CAD build for the part. Positions are in the model's coordinates, mm. Give positions to 0.01 mm unless a question says otherwise; leave off trailing zeros. Loops run counter-clockwise (first coordinate to the right, second up) from the corner with the lowest first, then second, coordinate; pieces in that order, holes last. Notation, with made-up numbers: (71.25, 10) - (105.25, 10) arc R28 cw to (105.25, 39) - close; hole circle Ø2 at (75, 70.5). An arc over 180 degrees is marked (long way). Return JSON: item names as keys, results as strings.
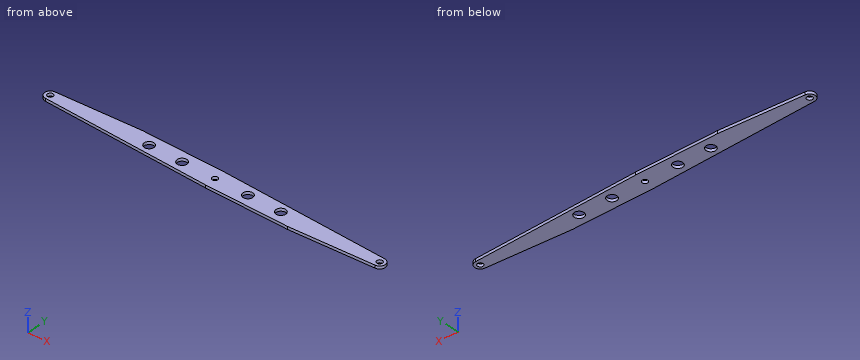
from build123d import *

# Parameters (mm, degrees)
SKETCH1_R           = 10
SKETCH1_R_2         = 17.5
BOSS_EXTRUDE1_DEPTH = 5


with BuildPart() as part:
    # Sketch1 → Boss-Extrude1 (new body, symmetric)
    with BuildSketch(Plane.XY):
        with BuildLine():
            Line((0, 40), (-300, 40))
            Line((-300, 40), (-601.327453078, 19.955898084))
            ThreePointArc((-601.327453078, 19.955898084), (-619.997257899, -0.331174458), (-600.665927363, -19.988910444))
            Line((-600.665927363, -19.988910444), (0, -40))
            Line((0, -40), (300, -40))
            Line((300, -40), (601.327453078, -19.955898084))
            ThreePointArc((601.327453078, -19.955898084), (619.997257899, 0.331174458), (600.665927363, 19.988910444))
            Line((600.665927363, 19.988910444), (0, 40))
        make_face()
        with Locations((-600, 0)):
            Circle(SKETCH1_R, mode=Mode.SUBTRACT)
        with Locations((600, 0)):
            Circle(SKETCH1_R, mode=Mode.SUBTRACT)
        Circle(SKETCH1_R, mode=Mode.SUBTRACT)
        with Locations((-120, 0)):
            Circle(SKETCH1_R_2, mode=Mode.SUBTRACT)
        with Locations((-240, 0)):
            Circle(SKETCH1_R_2, mode=Mode.SUBTRACT)
        with Locations((120, 0)):
            Circle(SKETCH1_R_2, mode=Mode.SUBTRACT)
        with Locations((240, 0)):
            Circle(SKETCH1_R_2, mode=Mode.SUBTRACT)
    extrude(amount=BOSS_EXTRUDE1_DEPTH, both=True)


solid = part.part
1. Drop flat-ended pins along their axis: P1, Ø4, axis at x = -422.5, z = -1.5, coming from the +Y side; P2, Ø3, axis at x = 333.5, z = 1, coming from the +Y side. Give the stop position or say it passes through.
Values follow:
{"P1": "stops at y = 31.98", "P2": "stops at y = 28.94"}
2. Cut at A-A, the plane z = -2.5. Write the cut outline in (x, y), plus the area to 3 significant figures.
Values follow:
{"outline": "(-601.33, 19.96) arc R20 ccw to (-600.67, -19.99) - (0, -40) - (300, -40) - (601.33, -19.96) arc R20 ccw to (600.67, 19.99) - (0, 40) - (-300, 40) - close; hole circle Ø20 at (-600, 0); hole circle Ø35 at (-240, 0); hole circle Ø35 at (-120, 0); hole circle Ø20 at (0, 0); hole circle Ø35 at (120, 0); hole circle Ø35 at (240, 0); hole circle Ø20 at (600, 0)", "area": "74,500 mm²"}
3. Cut at D-D, the plane x = -542. Write the cut outline in (y, z).
Values follow:
{"outline": "(-21.94, -5) - (23.9, -5) - (23.9, 5) - (-21.94, 5) - close"}
4. Cut at B-B, the plane x = 120. Write the cut outline in (y, z).
Values follow:
{"outline": "(-40, -5) - (-17.5, -5) - (-17.5, 5) - (-40, 5) - close; (17.5, -5) - (36, -5) - (36, 5) - (17.5, 5) - close"}
5. Drill centre lines: probe 1 along X at (y, z) = (11, -0.25); probe 2 along Y at (x, z) = (2, 3.25); probe 3 along X at (y, z) = (-11.5, -2.5). Where is each one in solid material? Low to high.
Values follow:
{"probe 1": "x = -616.7 to -253.61, -226.39 to -133.61, -106.39 to 106.39, 133.61 to 226.39, 253.61 to 616.7", "probe 2": "y = -40 to -9.8, 9.8 to 39.93", "probe 3": "x = -616.36 to -253.19, -226.81 to -133.19, -106.81 to 106.81, 133.19 to 226.81, 253.19 to 616.36"}
6. Cut at C-C, the plane y = 0. Give the number of separate pieces and of enclosed holes in the cut face, plus the area to 3 significant figures.
Values follow:
{"separate pieces": "8", "enclosed holes": "0", "area": "10,400 mm²"}
